Check sheet for the modelled part. Datum: model origin and axes. Units: mm. A direction names the side the tool comes from. Coordinates: 2 decimals unless noted, no trailing zeros. Order: outer loops, then holes, each group sorted by start corner. A loop starts at its lowest first (then second) coordinate and runs counter-clockwise, first axis right, second up.
from build123d import *

# Parameters (mm, degrees)
SKETCH1_W           = 21
SKETCH1_H           = 30
SKETCH1_R           = 1.75
BOSS_EXTRUDE1_DEPTH = 4
SKETCH2_W           = 21
SKETCH2_H           = 6.5
CUT_EXTRUDE1_DEPTH  = 1
SKETCH3_W           = 0.4
SKETCH3_H           = 6.5
BOSS_EXTRUDE2_DEPTH = 0.6


with BuildPart() as part:
    # Sketch1 → Boss-Extrude1 (new body)
    with BuildSketch(Plane.XY):
        with Locations((10.5, 15)):
            Rectangle(SKETCH1_W, SKETCH1_H)
        with Locations((4, 4)):
            Circle(SKETCH1_R, mode=Mode.SUBTRACT)
        with Locations((17, 4)):
            Circle(SKETCH1_R, mode=Mode.SUBTRACT)
        with Locations((17, 26)):
            Circle(SKETCH1_R, mode=Mode.SUBTRACT)
        with Locations((4, 26)):
            Circle(SKETCH1_R, mode=Mode.SUBTRACT)
    extrude(amount=BOSS_EXTRUDE1_DEPTH)

    # Sketch2 → Cut-Extrude1 (cut)
    with BuildSketch(Plane.XY.offset(4)):
        with Locations((10.5, 15)):
            Rectangle(SKETCH2_W, SKETCH2_H)
    extrude(amount=-CUT_EXTRUDE1_DEPTH, mode=Mode.SUBTRACT)

    # Sketch3 → Boss-Extrude2 (add)
    with BuildSketch(Plane.XY.offset(3)):
        with Locations((0.2, 15)):
            Rectangle(SKETCH3_W, SKETCH3_H)
        with Locations((1.2, 15)):
            Rectangle(SKETCH3_W, SKETCH3_H)
        with Locations((2.2, 15)):
            Rectangle(SKETCH3_W, SKETCH3_H)
        with Locations((3.2, 15)):
            Rectangle(SKETCH3_W, SKETCH3_H)
        with Locations((4.2, 15)):
            Rectangle(SKETCH3_W, SKETCH3_H)
        with Locations((5.2, 15)):
            Rectangle(SKETCH3_W, SKETCH3_H)
        with Locations((6.2, 15)):
            Rectangle(SKETCH3_W, SKETCH3_H)
        with Locations((7.2, 15)):
            Rectangle(SKETCH3_W, SKETCH3_H)
        with Locations((8.2, 15)):
            Rectangle(SKETCH3_W, SKETCH3_H)
        with Locations((9.2, 15)):
            Rectangle(SKETCH3_W, SKETCH3_H)
        with Locations((10.2, 15)):
            Rectangle(SKETCH3_W, SKETCH3_H)
        with Locations((11.2, 15)):
            Rectangle(SKETCH3_W, SKETCH3_H)
        with Locations((12.2, 15)):
            Rectangle(SKETCH3_W, SKETCH3_H)
        with Locations((13.2, 15)):
            Rectangle(SKETCH3_W, SKETCH3_H)
        with Locations((14.2, 15)):
            Rectangle(SKETCH3_W, SKETCH3_H)
        with Locations((15.2, 15)):
            Rectangle(SKETCH3_W, SKETCH3_H)
        with Locations((16.2, 15)):
            Rectangle(SKETCH3_W, SKETCH3_H)
        with Locations((17.2, 15)):
            Rectangle(SKETCH3_W, SKETCH3_H)
        with Locations((18.2, 15)):
            Rectangle(SKETCH3_W, SKETCH3_H)
        with Locations((19.2, 15)):
            Rectangle(SKETCH3_W, SKETCH3_H)
        with Locations((20.2, 15)):
            Rectangle(SKETCH3_W, SKETCH3_H)
    extrude(amount=BOSS_EXTRUDE2_DEPTH)


solid = part.part
(1) Tool access check on faces 4 (the flat face through (10.4, 18.25, 3.8)), 5 (the flat face through (10, 6, 4)). Record the directions out of +Z, -Z, +X, -X, +Y, -Y that give a thin tool (end or side, any length) a straight path to the whole face; none if there is none.
Filled in:
face 4: +Z
face 5: +Z, +X, -X, +Y, -Y
(2) Cross-section at B-B (z = 1.3). Enter the section's corners in (x, y).
Filled in:
outline: (0, 0) - (21, 0) - (21, 30) - (0, 30) - close; hole circle Ø3.5 at (4, 4); hole circle Ø3.5 at (4, 26); hole circle Ø3.5 at (17, 4); hole circle Ø3.5 at (17, 26)
(3) Cross-section at A-A (y = 4). Enter the section's corners in (x, z).
Filled in:
outline: (0, 0) - (2.25, 0) - (2.25, 4) - (0, 4) - close; (5.75, 0) - (15.25, 0) - (15.25, 4) - (5.75, 4) - close; (18.75, 0) - (21, 0) - (21, 4) - (18.75, 4) - close
(4) Go/stop test with a flat-tipped pin: P1, Ø0.5, axis at x = 6, y = 15, coming from the +Z side. Record where the tip stops, or that it passes through.
Filled in:
P1: stops at z = 3.6
(5) Thickness scan on probe 1 along Y at (x, z) = (17, 2.7); probe 2 along Y at (x, z) = (18, 1.65); probe 3 along Y at (x, z) = (13.5, 3.25). Record the ranges inside material, lowest first.
Filled in:
probe 1: y = 0 to 2.25, 5.75 to 24.25, 27.75 to 30
probe 2: y = 0 to 2.56, 5.44 to 24.56, 27.44 to 30
probe 3: y = 0 to 11.75, 18.25 to 30
(6) Release check for a two-part mould opening along X. For faces 1 (the cylindrical face through (16.62, 2.29, 1.97)), 2 (the flat face through (21, 15, 2)), 3 (the flat face through (10, 15, 0)) record: +X half, -X half, draft (parallel to the pull), parting line (faces both ways), or undercut.
Filled in:
face 1: undercut
face 2: +X half
face 3: draft
